Input: part model. Units: mm. Frame: model coordinates. Coordinates: 2 decimals unless noted, no trailing zeros. Loops run counter-clockwise (first coordinate to the right, second up) from the corner with the lowest first, then second, coordinate; pieces in that order, holes last.
Item 1: Section D-D on x = 9.5. Return loops of the section in (y, z), and give its area (3 significant figures).
Item 2: Section A-A on z = 0. Return loops of the section in (x, y), and give its area (3 significant figures).
Item 3: Ray query, line 1 along X through (y, z) = (0.6, 0); line 2 along Z through (x, y) = (-22.5, 0.2); line 3 along X through (y, z) = (0.8, 10). Return the intervals inside material, ascending.
Item 4: Section B-B on y = 0.2. Return loops of the section in (x, z), and give its area (3 significant figures).
Item 5: Section C-C on x = 0. Return loops of the section in (y, z).
Item 6: Contact query for flat-ended pins moving along their axis: P1, Ø12, axis at x = 2.5, z = 1, coming from the +Y side; P2, Ø3, axis at x = 20.5, z = -8.5, coming from the +Y side. Output: stop coordinate, or through.
```python
from build123d import *

# Parameters (mm, degrees)
SKETCH_1_R      = 13.5
SKETCH_1_R_2    = 4.5
EXTRUDE_1_DEPTH = 1


with BuildPart() as part:
    # 草圖1 → 伸長1 (new body)
    with BuildSketch(Plane(origin=(0, 0, 0), x_dir=(1, 0, 0), z_dir=(0, 1, 0))):
        with BuildLine():
            Line((18.973665961, 8), (22.5, 8))
            ThreePointArc((22.5, 8), (30.5, 0), (22.5, -8))
            Line((22.5, -8), (18.973665961, -8))
            ThreePointArc((18.973665961, -8), (18.439143477, -8.154845745), (18.070158058, -8.571428571))
            ThreePointArc((18.070158058, -8.571428571), (0, -20), (-18.070158058, -8.571428571))
            ThreePointArc((-18.070158058, -8.571428571), (-18.439143477, -8.154845745), (-18.973665961, -8))
            Line((-18.973665961, -8), (-22.5, -8))
            ThreePointArc((-22.5, -8), (-30.5, 0), (-22.5, 8))
            Line((-22.5, 8), (-18.973665961, 8))
            ThreePointArc((-18.973665961, 8), (-18.439143477, 8.154845745), (-18.070158058, 8.571428571))
            ThreePointArc((-18.070158058, 8.571428571), (0, 20), (18.070158058, 8.571428571))
            ThreePointArc((18.070158058, 8.571428571), (18.439143477, 8.154845745), (18.973665961, 8))
        make_face()
        with Locations(Location((0, 0, 0), (0, 0, 270))):
            Circle(SKETCH_1_R, mode=Mode.SUBTRACT)
        with Locations(Location((22.5, 0, 0), (0, 0, 270))):
            Circle(SKETCH_1_R_2, mode=Mode.SUBTRACT)
        with Locations(Location((-22.5, 0, 0), (0, 0, 90))):
            Circle(SKETCH_1_R_2, mode=Mode.SUBTRACT)
    extrude(amount=EXTRUDE_1_DEPTH)


solid = part.part
```
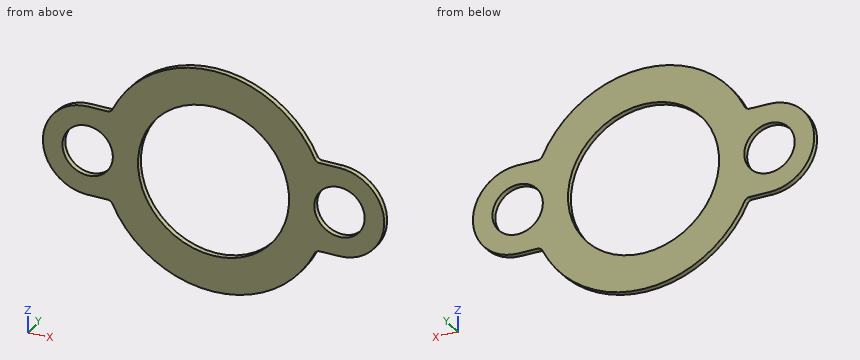
Results found:
1. outline: (0, -17.6) - (1, -17.6) - (1, -9.59) - (0, -9.59) - close; (0, 9.59) - (1, 9.59) - (1, 17.6) - (0, 17.6) - close
1. area: 16.0 mm2
2. outline: (-30.5, 0) - (-27, 0) - (-27, 1) - (-30.5, 1) - close; (-18, 0) - (-13.5, 0) - (-13.5, 1) - (-18, 1) - close; (13.5, 0) - (18, 0) - (18, 1) - (13.5, 1) - close; (27, 0) - (30.5, 0) - (30.5, 1) - (27, 1) - close
2. area: 16.0 mm2
3. line 1: x = -30.5 to -27, -18 to -13.5, 13.5 to 18, 27 to 30.5
3. line 2: z = -8 to -4.5, 4.5 to 8
3. line 3: x = -17.32 to -9.07, 9.07 to 17.32
4. outline: (-22.5, -8) - (-18.97, -8) arc R1 cw to (-18.07, -8.57) arc R20 ccw to (18.07, -8.57) arc R1 cw to (18.97, -8) - (22.5, -8) arc R8 ccw to (22.5, 8) - (18.97, 8) arc R1 cw to (18.07, 8.57) arc R20 ccw to (-18.07, 8.57) arc R1 cw to (-18.97, 8) - (-22.5, 8) arc R8 ccw to start; hole circle Ø9 at (-22.5, 0); hole circle Ø27 at (0, 0); hole circle Ø9 at (22.5, 0)
4. area: 856 mm2
5. outline: (0, -20) - (1, -20) - (1, -13.5) - (0, -13.5) - close; (0, 13.5) - (1, 13.5) - (1, 20) - (0, 20) - close
6. P1: passes through
6. P2: stops at y = 1
